Can you work these out from the model? Positions are in its coordinate system, mm. A direction names the side the tool comes from. Give positions to 0.01 mm unless a question says otherwise; leave off trailing zeros. Loops run counter-clockwise (first coordinate to the right, second up) from the corner with the lowest first, then second, coordinate; pieces in that order, holes last. Notation, with made-up numbers: (41, 71.5) - (95, 71.5) arc R18 cw to (95, 96.5) - close; hole circle Ø7 at (78, -36.75). An arc over 180 degrees is marked (long way). Answer as a JSON object with one key per item and string values. Group by question number.
Item 1: Thinking about a two-plate mould opening in Z: for faces 1 (the cylindrical face through (-57.916, -0.112, 17.245)), 2 (the cylindrical face through (-6, 0, 5)), 3 (the cylindrical face through (-117.37, 0.11, 28.76)), which applies, pulls with the +Z half, pulls with the -Z half, needs draft (parallel to the pull), parting line crosses it, or undercut?
Item 2: Suppose I cut it at D-D on z = 14. Write out the boundary of the cut face in (x, y), and give its area (3 significant figures).
Item 3: Will these pins go through, and if not, where does the flat tip stop? pin 1 (11 mm diameter, centred on y = -16.5, z = 4, fed in from -X); pin 2 (15.5 mm diameter, centred on x = 0, y = 0, fed in from +Z); pin 3 (1.5 mm diameter, centred on y = -32, z = 9.5, fed in from -X).
Item 4: Suppose I cut it at B-B on y = -21.5. Write out the boundary of the cut face in (x, z).
Item 5: Which directions (+Z, -Z, +X, -X, +Y, -Y) give clear straight access to the entire face, cutting with the end or side of a thin tool? Please do faces 4 (the flat face through (-68, -16, 5)), 5 (the flat face through (-68, 17, 5)), 6 (the cylindrical face through (-19.61, 22.84, 4.93)), 7 (the flat face through (-35, 12, 10)).
Item 6: Suppose I cut it at A-A on y = 0. Write out the boundary of the cut face in (x, z), and give its area (3 significant figures).
Item 7: Please list where these lines run through material, in increasing order: L1, parallel to Y at x = -50, z = 7; L2, parallel to Z at x = -41, y = -26.5; L3, parallel to Y at x = -98.5, z = 37.5.
Item 8: Suppose I cut it at C-C on x = -50. Write out the boundary of the cut face in (y, z).
from build123d import *

# Parameters (mm, degrees)
F0_R          = 6
F1_DEPTH      = 10
F2_R          = 10
F3_DEPTH      = 8
F3_DEPTH_BACK = 8


with BuildPart() as f1:
    # F0 (on Top) → F1 (new body)
    with BuildSketch(Plane.XY):
        with BuildLine():
            ThreePointArc((-34.676423, -32.725742), (-20.892766, -20.461597), (-2.634981, -17.806091))
            ThreePointArc((-2.634981, -17.806091), (17.951457, -1.321053), (0, 18))
            ThreePointArc((0, 18), (-19.862144, 22.974), (-35.035837, 36.721888))
            ThreePointArc((-35.035837, 36.721888), (-55.227096, 43.942524), (-68, 26.718197))
            Line((-68, 26.718197), (-68, -23.281803))
            ThreePointArc((-68, -23.281803), (-54.907933, -40.599777), (-34.676423, -32.725742))
        make_face()
        with Locations((-50, -23.281803)):
            Circle(F0_R, mode=Mode.SUBTRACT)
        Circle(F0_R, mode=Mode.SUBTRACT)
        with Locations((-50, 26.718197)):
            Circle(F0_R, mode=Mode.SUBTRACT)
    extrude(amount=F1_DEPTH)

    # F2 (on Front) → F3 (join, two sides)
    with BuildSketch(Plane.XZ) as f3_sk:
        with BuildLine():
            ThreePointArc((-15.978726, 10), (-58.487228, 17.449895), (-95.928789, 38.911565))
            ThreePointArc((-95.928789, 38.911565), (-130.688818, 29.481496), (-110, 0))
            Line((-110, 0), (-15.978726, 0))
            Line((-15.978726, 0), (-15.978726, 10))
        make_face()
        with Locations((-110, 22)):
            Circle(F2_R, mode=Mode.SUBTRACT)
    extrude(amount=F3_DEPTH)
    extrude(f3_sk.sketch, amount=-F3_DEPTH_BACK)


solid = f1.part
Worked out:
{
 "1": {"face 1": "pulls with the +Z half", "face 2": "needs draft", "face 3": "undercut"},
 "2": {"outline": "(-130.49, -8) - (-116, -8) - (-116, 8) - (-130.49, 8) - close; (-104, -8) - (-47.35, -8) - (-47.35, 8) - (-104, 8) - close", "area": "1,140 mm2"},
 "3": {"pin 1": "stops at x = -68", "pin 2": "stops at z = 10", "pin 3": "stops at x = -66.14"},
 "4": {"outline": "(-68, 0) - (-55.73, 0) - (-55.73, 10) - (-68, 10) - close; (-44.27, 0) - (-22.93, 0) - (-22.93, 10) - (-44.27, 10) - close"},
 "5": {"face 4": "+Z, -Z, -X, -Y", "face 5": "+Z, -Z, -X, +Y", "face 6": "+Z, -Z, +X, +Y", "face 7": "+Z, +X"},
 "6": {"outline": "(-110, 0) - (-6, 0) - (-6, 10) - (-15.98, 10) arc R125 cw to (-95.93, 38.91) arc R22 ccw (long way) to start; (6, 0) - (18, 0) - (18, 10) - (6, 10) - close; hole circle Ø20 at (-110, 22)", "area": "2,790 mm2"},
 "7": {"L1": "y = -41.28 to -29.28, -17.28 to 20.72, 32.72 to 44.72", "L2": "z = 0 to 10", "L3": "y = -8 to 8"},
 "8": {"outline": "(-41.28, 0) - (-29.28, 0) - (-29.28, 10) - (-41.28, 10) - close; (-17.28, 0) - (20.72, 0) - (20.72, 10) - (8, 10) - (8, 14.72) - (-8, 14.72) - (-8, 10) - (-17.28, 10) - close; (32.72, 0) - (44.72, 0) - (44.72, 10) - (32.72, 10) - close"}
}
